```python
from build123d import *

# Parameters (mm, degrees)
SKETCH1_R           = 25
BOSS_EXTRUDE1_DEPTH = 110
SKETCH2_OUTSIDE_W   = 78.154
SKETCH2_OUTSIDE_H   = 78.154
SKETCH2_OUTSIDE_W_2 = 24
SKETCH2_OUTSIDE_H_2 = 24
CUT_EXTRUDE1_DEPTH  = 45
SKETCH3_OUTSIDE_W   = 78.154
SKETCH3_OUTSIDE_H   = 78.154
SKETCH3_OUTSIDE_R   = 12
CUT_EXTRUDE2_DEPTH  = 20
SKETCH4_OUTSIDE_W   = 78.154
SKETCH4_OUTSIDE_H   = 78.154
SKETCH4_OUTSIDE_R   = 15
CUT_EXTRUDE3_DEPTH  = 33
CHAMFER1_SIZE       = 2
SKETCH5_W           = 20
SKETCH5_H           = 16
CUT_EXTRUDE4_DEPTH  = 2
CUT_EXTRUDE5_DEPTH  = 5


with BuildPart() as part:
    # Sketch1 → Boss-Extrude1 (new body)
    with BuildSketch(Plane(origin=(0, 0, 0), x_dir=(0, 0, -1), z_dir=(1, 0, 0))):
        Circle(SKETCH1_R)
    extrude(amount=BOSS_EXTRUDE1_DEPTH)

    # Sketch2 outside → Cut-Extrude1 (cut)
    with BuildSketch(Plane(origin=(110, 0, 0), x_dir=(0, 0, -1), z_dir=(1, 0, 0))):
        Rectangle(SKETCH2_OUTSIDE_W, SKETCH2_OUTSIDE_H)
        Rectangle(SKETCH2_OUTSIDE_W_2, SKETCH2_OUTSIDE_H_2, mode=Mode.SUBTRACT)
    extrude(amount=-CUT_EXTRUDE1_DEPTH, mode=Mode.SUBTRACT)

    # Sketch3 outside → Cut-Extrude2 (cut)
    with BuildSketch(Plane(origin=(110, 0, 0), x_dir=(0, 0, -1), z_dir=(1, 0, 0))):
        Rectangle(SKETCH3_OUTSIDE_W, SKETCH3_OUTSIDE_H)
        Circle(SKETCH3_OUTSIDE_R, mode=Mode.SUBTRACT)
    extrude(amount=-CUT_EXTRUDE2_DEPTH, mode=Mode.SUBTRACT)

    # Sketch4 outside → Cut-Extrude3 (cut)
    with BuildSketch(Plane.ZY):
        Rectangle(SKETCH4_OUTSIDE_W, SKETCH4_OUTSIDE_H)
        Circle(SKETCH4_OUTSIDE_R, mode=Mode.SUBTRACT)
    extrude(amount=-CUT_EXTRUDE3_DEPTH, mode=Mode.SUBTRACT)

    # Chamfer1
    chamfer1_edges = [part.edges().sort_by_distance(p)[0] for p in [
        (0, 0, -15),
    ]]
    chamfer(chamfer1_edges, length=CHAMFER1_SIZE)

    # Sketch5 → Cut-Extrude4 (cut)
    with BuildSketch(Plane(origin=(0, 15, 0), x_dir=(1, 0, 0), z_dir=(0, 1, 0))):
        with Locations((10, 0)):
            Rectangle(SKETCH5_W, SKETCH5_H)
    extrude(amount=-CUT_EXTRUDE4_DEPTH, mode=Mode.SUBTRACT)

    # Sketch6 → Cut-Extrude5 (cut)
    with BuildSketch(Plane(origin=(0, 25, 0), x_dir=(1, 0, 0), z_dir=(0, 1, 0))):
        with BuildLine():
            Line((44, -5), (54, -5))
            ThreePointArc((54, -5), (59, 0), (54, 5))
            Line((54, 5), (44, 5))
            ThreePointArc((44, 5), (39, 0), (44, -5))
        make_face()
    extrude(amount=-CUT_EXTRUDE5_DEPTH, mode=Mode.SUBTRACT)


solid = part.part
```
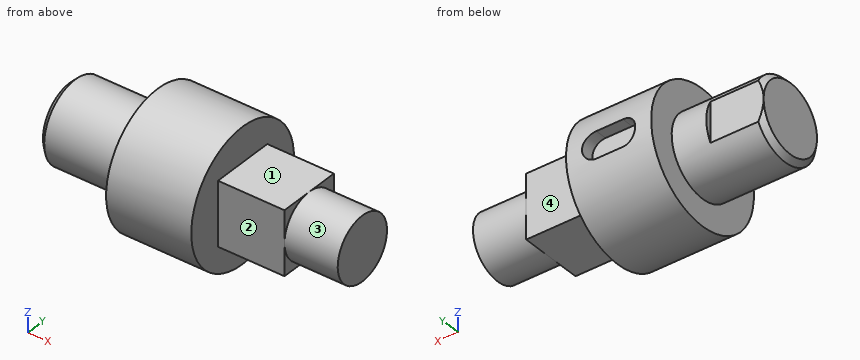
Here's how the part is built. I have some questions about the finished solid (model axes, mm). Face numbers are marked on the shaded views. A direction names the side the tool comes from. Round coordinates to 2 decimals unless told otherwise and drop trailing zeros. Write each loop counter-clockwise with the first axis right and the second up, starting at its lowest first coordinate (ties: lowest second). Pieces come first, ordered by that corner, then holes.
Q1. If we section it at C-C on z = -21: Write out the boundary of the cut face in (x, y), plus the area to 3 significant figures.
Q2. Will these pins go through, and if not, where does the flat tip stop? P1, Ø5, axis at y = 15, z = -14.5, coming from the +X side; P2, Ø1.3, axis at x = 46.5, y = 22.5, coming from the -Z side; P3, Ø6, axis at x = 35, z = 10, coming from the +Y side.
Q3. Which directions (+Z, -Z, +X, -X, +Y, -Y) give clear straight access to the entire face, cutting with the end or side of a thin tool? Please do the marked faces 1, 2, 3 and 4.
Q4. If we section it at A-A on y = 21.5: Write out the boundary of the cut face in (x, z).
Q5. Please list where these lines run through material, in increasing order: probe 1 along X at (y, z) = (19, 5.5); probe 2 along Z at (x, y) = (30.5, 0.5); probe 3 along Z at (x, y) = (18.5, 9).
Q6. If we section it at D-D on x = 80.5: Write out the boundary of the cut face in (y, z).
Q7. If we section it at B-B on x = 36: Write out the boundary of the cut face in (y, z), plus the area to 3 significant figures.
Answer below:
1. outline: (33, -13.56) - (65, -13.56) - (65, 13.56) - (33, 13.56) - close
1. area: 868 mm2
2. P1: stops at x = 65
2. P2: stops at z = -12.15
2. P3: stops at y = 24
3. face 1: +Z, +X, +Y, -Y
3. face 2: +Z, -Z, +X, -Y
3. face 3: +X
3. face 4: +Z, -Z, +X, +Y
4. outline: (33, -12.76) - (65, -12.76) - (65, 12.76) - (33, 12.76) - close; hole (44, -5) - (54, -5) arc R5 ccw to (54, 5) - (44, 5) arc R5 ccw to start
5. probe 1: x = 33 to 65
5. probe 2: z = -14.99 to 14.99
5. probe 3: z = -12 to 12
6. outline: (-12, -12) - (12, -12) - (12, 12) - (-12, 12) - close
7. outline: circle Ø50 at (0, 0)
7. area: 1,960 mm2
